Could you check a few things on this model? Use its own coordinates, in mm. Face numbers are marked on the shaded views. A direction names the side the tool comes from. Round coordinates to 2 decimals unless told otherwise and drop trailing zeros. Loops run counter-clockwise (first coordinate to the right, second up) from the corner with the lowest first, then second, coordinate; pieces in that order, holes last. Notation, with made-up numbers: (19.25, 28.5) -> (39.25, 28.5) arc R18 ccw to (39.25, 49.5) -> close; hole circle Ø7 at (82, 71). An arc over 180 degrees is marked (long way). One line per item, written item: value.
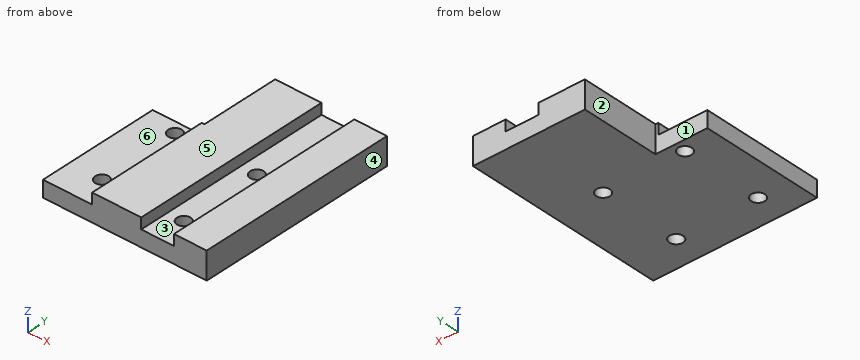
```python
from build123d import *

# Parameters (mm, degrees)
BOSS_EXTRUDE1_DEPTH      = 6
SKETCH2_W                = 12
SKETCH2_H                = 74
SKETCH2_W_2              = 1
SKETCH2_H_2              = 45
BOSS_EXTRUDE2_DEPTH      = 4
F_5_0_5_DIAMETER_HOLE1_D = 5
F_5_0_5_DIAMETER_HOLE2_D = 5


with BuildPart() as part:
    # Sketch1 → Boss-Extrude1 (new body)
    with BuildSketch(Plane.XY):
        Polygon((0, 0), (0, 45), (19, 45), (19, 74), (60, 74), (60, 0), align=None)
    extrude(amount=BOSS_EXTRUDE1_DEPTH)

    # Sketch2 → Boss-Extrude2 (add)
    with BuildSketch(Plane.XY.offset(6)):
        Polygon((36, 0), (36, 74), (19, 74), (19, 45), (19, 0), align=None)
        with Locations((54, 37)):
            Rectangle(SKETCH2_W, SKETCH2_H)
        with Locations((18.5, 22.5)):
            Rectangle(SKETCH2_W_2, SKETCH2_H_2)
    extrude(amount=BOSS_EXTRUDE2_DEPTH)

    # Ø5.0 (5) Diameter Hole1 (through all)
    with Locations(Plane.XY.offset(6)):
        with Locations((42, 40.75), (42, 10.75)):
            Hole(F_5_0_5_DIAMETER_HOLE1_D / 2)

    # Ø5.0 (5) Diameter Hole2 (through all)
    with Locations(Plane.XY.offset(6)):
        with Locations((12, 10.75), (12, 40.75)):
            Hole(F_5_0_5_DIAMETER_HOLE2_D / 2)


solid = part.part
```
(1) Imagine slicing it at A-A on x = 12. Write out the boundary of the cut face in (y, z), then the cut area to 3 significant figures.
Results below:
outline: (0, 0) -> (8.25, 0) -> (8.25, 6) -> (0, 6) -> close; (13.25, 0) -> (38.25, 0) -> (38.25, 6) -> (13.25, 6) -> close; (43.25, 0) -> (45, 0) -> (45, 6) -> (43.25, 6) -> close
area: 210 mm²
(2) For pin 1 Ø6 at (x, y) = (12, 40.75) entering from +Z, with a flat end and sliding along its axis, tell me the tip position at first contact or that it passes through.
Results below:
pin 1: stops at z = 6
(3) Imagine slicing it at D-D on x = 42. Write out the boundary of the cut face in (y, z), then the cut area to 3 significant figures.
Results below:
outline: (0, 0) -> (8.25, 0) -> (8.25, 6) -> (0, 6) -> close; (13.25, 0) -> (38.25, 0) -> (38.25, 6) -> (13.25, 6) -> close; (43.25, 0) -> (74, 0) -> (74, 6) -> (43.25, 6) -> close
area: 384 mm²
(4) Imagine slicing it at C-C on z = 4. Write out the boundary of the cut face in (x, y).
Results below:
outline: (0, 0) -> (60, 0) -> (60, 74) -> (19, 74) -> (19, 45) -> (0, 45) -> close; hole circle Ø5 at (12, 10.75); hole circle Ø5 at (12, 40.75); hole circle Ø5 at (42, 10.75); hole circle Ø5 at (42, 40.75)
(5) On a 3-axis mill with a long thin cutter (end or side, diameter ignored), from which of +Z, -Z, +X, -X, +Y, -Y can I reach the whole of each face in a straight line? I mean the marked faces 5 and 6. Say none if no direction works.
Results below:
face 5: +Z, +X, -X, +Y, -Y
face 6: +Z, -X, +Y, -Y
(6) We'd pull the mould along X, two halves only. Please class the marked faces 1, 2, 3 and 4: +X half, -X half, draft (parallel to the pull), parting line (faces both ways), or undercut.
Results below:
face 1: draft
face 2: -X half
face 3: undercut
face 4: +X half
(7) Please list where these lines run through material, in increasing order: L1, parallel to Y at x = 12, z = 4.5; L2, parallel to X at y = 26.5, z = 8; L3, parallel to Y at x = 42, z = 4.5.
Results below:
L1: y = 0 to 8.25, 13.25 to 38.25, 43.25 to 45
L2: x = 18 to 36, 48 to 60
L3: y = 0 to 8.25, 13.25 to 38.25, 43.25 to 74
(8) Imagine slicing it at B-B on y = 10.75. Write out the boundary of the cut face in (x, z).
Results below:
outline: (0, 0) -> (9.5, 0) -> (9.5, 6) -> (0, 6) -> close; (14.5, 0) -> (39.5, 0) -> (39.5, 6) -> (36, 6) -> (36, 10) -> (18, 10) -> (18, 6) -> (14.5, 6) -> close; (44.5, 0) -> (60, 0) -> (60, 10) -> (48, 10) -> (48, 6) -> (44.5, 6) -> close
